from build123d import *

# Parameters (mm, degrees)
SKETCH1_R           = 56
BOSS_EXTRUDE1_DEPTH = 3
FILLET1_R           = 10
SKETCH2_R           = 2.6
SKETCH2_R_2         = 1.6
CUT_EXTRUDE1_DEPTH  = 482.049893462


with BuildPart() as part:
    # Sketch1 → Boss-Extrude1 (new body)
    with BuildSketch(Plane(origin=(0, 0, 0), x_dir=(1, 0, 0), z_dir=(0, 1, 0))):
        Polygon((70, 100), (70, 0), (260, 0), (260, 100), (330, 100), (330, 250), (260, 250), (260, 350), (70, 350), (70, 250), (0, 250), (0, 100), align=None)
        with Locations(Location((165, 100, 0), (0, 0, 270))):
            Circle(SKETCH1_R, mode=Mode.SUBTRACT)
    extrude(amount=BOSS_EXTRUDE1_DEPTH)

    # Fillet1
    fillet1_edges = [part.edges().sort_by_distance(p)[0] for p in [
        (70, 1.5, 0),
        (70, 1.5, -100),
        (0, 1.5, -100),
        (0, 1.5, -250),
        (70, 1.5, -250),
        (70, 1.5, -350),
        (260, 1.5, -350),
        (260, 1.5, -250),
        (330, 1.5, -250),
        (330, 1.5, -100),
        (260, 1.5, -100),
        (260, 1.5, 0),
    ]]
    fillet(fillet1_edges, radius=FILLET1_R)

    # Sketch2 → Cut-Extrude1 (cut, through all)
    with BuildSketch(Plane(origin=(0, 3, 0), x_dir=(1, 0, 0), z_dir=(0, 1, 0))):
        with Locations(Location((100, 340, 0), (0, 0, 270))):
            Circle(SKETCH2_R)
        with Locations(Location((135, 340, 0), (0, 0, 270))):
            Circle(SKETCH2_R)
        with Locations(Location((195, 340, 0), (0, 0, 270))):
            Circle(SKETCH2_R)
        with Locations(Location((230, 340, 0), (0, 0, 270))):
            Circle(SKETCH2_R)
        with Locations(Location((10, 220, 0), (0, 0, 270))):
            Circle(SKETCH2_R)
        with Locations(Location((10, 185, 0), (0, 0, 270))):
            Circle(SKETCH2_R)
        with Locations(Location((10, 130, 0), (0, 0, 270))):
            Circle(SKETCH2_R)
        with Locations(Location((10, 165, 0), (0, 0, 270))):
            Circle(SKETCH2_R)
        with Locations(Location((100, 10, 0), (0, 0, 270))):
            Circle(SKETCH2_R)
        with Locations(Location((135, 10, 0), (0, 0, 270))):
            Circle(SKETCH2_R)
        with Locations(Location((195, 10, 0), (0, 0, 270))):
            Circle(SKETCH2_R)
        with Locations(Location((230, 10, 0), (0, 0, 270))):
            Circle(SKETCH2_R)
        with Locations(Location((320, 130, 0), (0, 0, 270))):
            Circle(SKETCH2_R)
        with Locations(Location((320, 165, 0), (0, 0, 270))):
            Circle(SKETCH2_R)
        with Locations(Location((320, 220, 0), (0, 0, 270))):
            Circle(SKETCH2_R)
        with Locations(Location((320, 185, 0), (0, 0, 270))):
            Circle(SKETCH2_R)
        with Locations(Location((165, 165, 0), (0, 0, 270))):
            Circle(SKETCH2_R_2)
        with Locations(Location((210.961940777, 145.961940777, 0), (0, 0, 270))):
            Circle(SKETCH2_R_2)
        with Locations(Location((230, 100, 0), (0, 0, 270))):
            Circle(SKETCH2_R_2)
        with Locations(Location((210.961940777, 54.038059223, 0), (0, 0, 270))):
            Circle(SKETCH2_R_2)
        with Locations(Location((165, 35, 0), (0, 0, 270))):
            Circle(SKETCH2_R_2)
        with Locations(Location((119.038059223, 54.038059223, 0), (0, 0, 270))):
            Circle(SKETCH2_R_2)
        with Locations(Location((100, 100, 0), (0, 0, 270))):
            Circle(SKETCH2_R_2)
        with Locations(Location((119.038059223, 145.961940777, 0), (0, 0, 270))):
            Circle(SKETCH2_R_2)
    extrude(amount=-CUT_EXTRUDE1_DEPTH, mode=Mode.SUBTRACT)


solid = part.part
Work out the finished part from the listing and answer in its coordinate system (mm). Give positions to 0.01 mm unless a question says otherwise; leave off trailing zeros. Write each loop counter-clockwise with the first axis right and the second up, starting at its lowest first coordinate (ties: lowest second). Pieces come first, ordered by that corner, then holes. Notation, with made-up numbers: M -2,49 L 8,49 A21 ccw 8,72 Z; hole C 54,-11.75 d7. An arc over 180 degrees is marked long. Answer as CSV lines item,"result".
Q1. The mould has two halves that part along X. Classify faces 1 (the cylindrical face through (256.99, 1.52, -2.85)), 2 (the cylindrical face through (66.99, 1.52, -252.85)), 3 (the cylindrical face through (110.33, 1.48, -112.14)), 4 (the flat face through (163, 3, -177)): +X half, -X half, draft (parallel to the pull), parting line (faces both ways), or undercut.
A:
face 1,"+X half"
face 2,"-X half"
face 3,"undercut"
face 4,"draft"
Q2. Given P1, Ø4.5, axis at x = 100, z = -10, coming from the -Y side; P2, Ø0.9, axis at y = 1, z = -303.5, coming from the +X side; P3, Ø0.9, axis at y = 2, z = -295.5, coming from the -X side, each flat-ended and moving along its own axis, determine where each tip first touches the part or whether it passes through.
A:
P1,"passes through"
P2,"stops at x = 260"
P3,"stops at x = 70"
Q3. A cutting plane is placed at C-C on z = -270. Write down the section's boundary in (x, y).
A:
outline,"M 70,0 L 260,0 L 260,3 L 70,3 Z"
Q4. A cutting plane is placed at A-A on z = -139. Write down the section's boundary in (x, y).
A:
outline,"M 0,0 L 124.81,0 L 124.81,3 L 0,3 Z; M 205.19,0 L 330,0 L 330,3 L 205.19,3 Z"
Q5. Find the intervals of material crossed by probe 1 along Z at (x, y) = (320, 1.25); probe 2 along X at (y, z) = (0.7, -165); probe 3 along X at (y, z) = (0.8, -340), in increasing order. Write a range as [from, to].
A:
probe 1,"z = [-250, -222.6], [-217.4, -187.6], [-182.4, -167.6], [-162.4, -132.6], [-127.4, -100]"
probe 2,"x = [0, 7.4], [12.6, 163.4], [166.6, 317.4], [322.6, 330]"
probe 3,"x = [70, 97.4], [102.6, 132.4], [137.6, 192.4], [197.6, 227.4], [232.6, 260]"
Q6. A cutting plane is placed at D-D on y = 1.2. Count the separate pieces of the cut face and the enclosed holes in it, plus the area to 3 significant figures.
A:
separate pieces,"1"
enclosed holes,"25"
area,"77,200 mm²"
Q7. A cutting plane is placed at B-B on x = 49. Write down the section's boundary in (y, z).
A:
outline,"M 0,-250 L 3,-250 L 3,-100 L 0,-100 Z"
